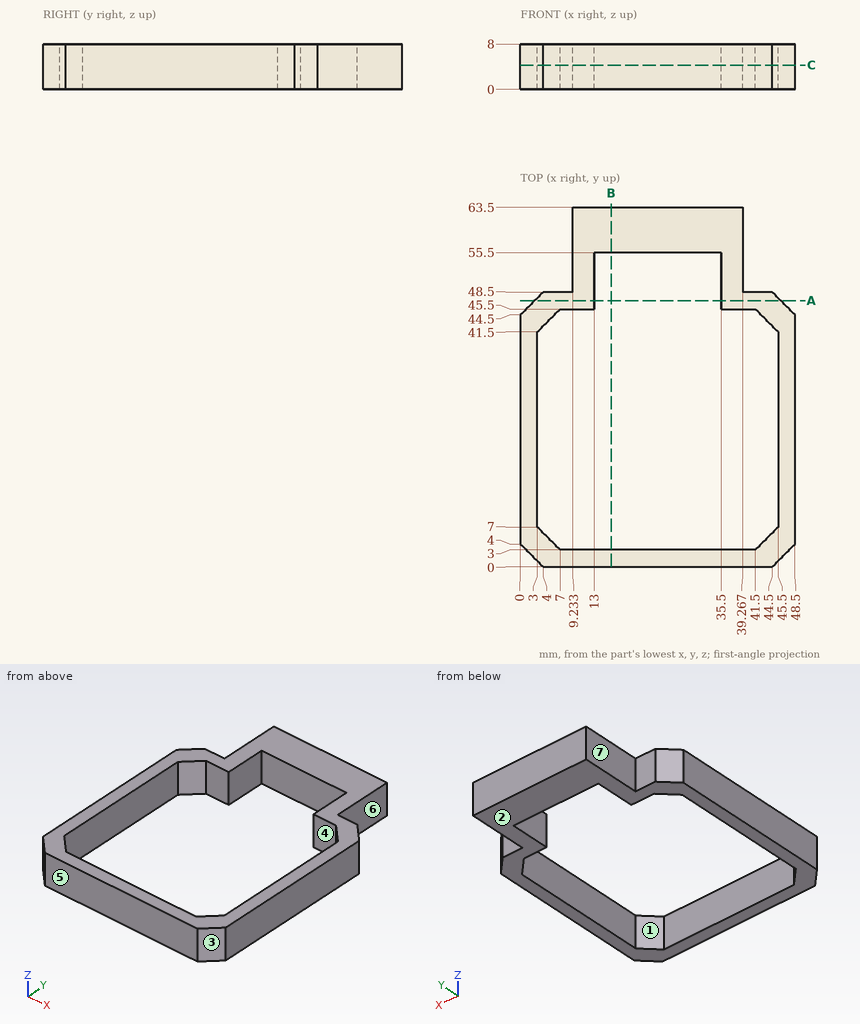
The figure shows three views and two pictorial views of one solid part (mm, origin at its lowest corner). Answer the questions. A direction names the side the tool comes from. Give positions to 0.01 mm unless a question says otherwise; leave off trailing zeros. Write each loop counter-clockwise with the first axis right and the second up, starting at its lowest first coordinate (ties: lowest second). Pieces come first, ordered by that corner, then holes. Notation, with made-up numbers: (-2, -24) - (6, -24) arc R21 cw to (6, -6) - close; hole circle Ø6 at (79.25, 27). An arc over 180 degrees is marked (long way). Use one line per item in the form item = value.
1. A cutting plane is placed at A-A (y = 47). Write down the section's boundary in (x, z), and give its area (3 significant figures).
Filled in:
outline = (2.5, 0) - (13, 0) - (13, 8) - (2.5, 8) - close; (35.5, 0) - (46, 0) - (46, 8) - (35.5, 8) - close
area = 168 mm^2
2. A cutting plane is placed at C-C (z = 4.25). Write down the section's boundary in (x, y).
Filled in:
outline = (0, 4) - (4, 0) - (44.5, 0) - (48.5, 4) - (48.5, 44.5) - (44.5, 48.5) - (39.27, 48.5) - (39.27, 63.5) - (9.23, 63.5) - (9.23, 48.5) - (4, 48.5) - (0, 44.5) - close; hole (3, 7) - (7, 3) - (41.5, 3) - (45.5, 7) - (45.5, 41.5) - (41.5, 45.5) - (35.5, 45.5) - (35.5, 55.5) - (13, 55.5) - (13, 45.5) - (7, 45.5) - (3, 41.5) - close
3. Each of these flat-tipped pins is pushed along its axis until it touches: pin 1 Ø4 at (y, z) = (51, 6) entering from -X; pin 2 Ø3 at (x, z) = (42, 2) entering from -Y; pin 3 Ø1.6 at (x, z) = (41, 5) entering from +Y; pin 4 Ø6 at (x, y) = (8, 36) entering from -Z. Where does it stop, or does it pass through?
Filled in:
pin_1 = 9.23
pin_2 = 0
pin_3 = 48.5
pin_4 = through
4. For the marked faces 4, 5, 6 and 7, determine the directions among +Z, -Z, +X, -X, +Y, -Y from which every point of the face is accessible in a straight line to the end or side of a thin tool.
Filled in:
face_4 = +Z, -Z
face_5 = +Z, -Z, +X, -X, -Y
face_6 = +Z, -Z, +X, +Y
face_7 = +Z, -Z, -X, +Y
5. Consider L1, parallel to X at y = 50, z = 4.5; L2, parallel to X at y = 18, z = 1.75; L3, parallel to Y at x = 6, z = 7. Determine where each line is inside the solid, lowest interval first.
Filled in:
L1 = 9.23 to 13, 35.5 to 39.27
L2 = 0 to 3, 45.5 to 48.5
L3 = 0 to 4, 44.5 to 48.5
6. A cutting plane is placed at B-B (x = 16). Write down the section's boundary in (y, z).
Filled in:
outline = (0, 0) - (3, 0) - (3, 8) - (0, 8) - close; (55.5, 0) - (63.5, 0) - (63.5, 8) - (55.5, 8) - close
7. Determine the mould class of the marked faces 1, 2 and 3 for opening direction X: released by +X, released by -X, zero draft, split by the parting line, or undercut.
Filled in:
face_1 = undercut
face_2 = zero draft
face_3 = released by +X
